CAD build for the part. Positions are in the model's coordinates, mm. A direction names the side the tool comes from. Give positions to 0.01 mm unless a question says otherwise; leave off trailing zeros. Loops run counter-clockwise (first coordinate to the right, second up) from the corner with the lowest first, then second, coordinate; pieces in that order, holes last. Notation, with made-up numbers: M 24,-14.5 L 28,-14.5 A25 ccw 28,13.5 Z; hole C 56.25,74.5 d4. An arc over 180 degrees is marked long. One line per question, with ' | ' between items.
```python
from build123d import *

# Parameters (mm, degrees)
BOSS_EXTRUDE1_DEPTH = 20
SKETCH5_W           = 9
SKETCH5_H           = 1.454272164
CUT_EXTRUDE4_DEPTH  = 10
SKETCH6_R           = 0.5
CUT_EXTRUDE5_DEPTH  = 5
CUT_EXTRUDE6_DEPTH  = 21
SKETCH11_R          = 1
CUT_EXTRUDE7_DEPTH  = 5


with BuildPart() as part:
    # Sketch1 → Boss-Extrude1 (new body)
    with BuildSketch(Plane.XY):
        with BuildLine():
            Line((0, 42.801960973), (0, -42.801960973))
            ThreePointArc((0, -42.801960973), (3.660110944, -50.535382386), (11.961161351, -52.60776773))
            Line((11.961161351, -52.60776773), (41.961161351, -46.60776773))
            ThreePointArc((41.961161351, -46.60776773), (47.733421413, -43.141850029), (50, -36.801960973))
            Line((50, -36.801960973), (50, 36.801960973))
            ThreePointArc((50, 36.801960973), (47.733421413, 43.141850029), (41.961161351, 46.60776773))
            Line((41.961161351, 46.60776773), (11.961161351, 52.60776773))
            ThreePointArc((11.961161351, 52.60776773), (3.660110944, 50.535382386), (0, 42.801960973))
        make_face()
    extrude(amount=BOSS_EXTRUDE1_DEPTH)

    # Sketch5 → Cut-Extrude4 (cut)
    with BuildSketch(Plane.ZY):
        with Locations((10, 16.569972364)):
            Rectangle(SKETCH5_W, SKETCH5_H)
    extrude(amount=-CUT_EXTRUDE4_DEPTH, mode=Mode.SUBTRACT)

    # Sketch6 → Cut-Extrude5 (cut)
    with BuildSketch(Plane.XZ.offset(-17.297108446)):
        with Locations((2.644871575, 10)):
            Circle(SKETCH6_R)
    extrude(amount=-CUT_EXTRUDE5_DEPTH, mode=Mode.SUBTRACT)

    # Sketch9 → Cut-Extrude6 (cut, through all)
    with BuildSketch(Plane.XY.offset(20)):
        Polygon((42.2, 5.497108446), (42.2, -10.402891554), (50, -10.402891554), (50, 12.297108446), (42.2, 12.297108446), (42.2, 7.997108446), (37.17, 7.997108446), (37.17, 5.497108446), align=None)
    extrude(amount=-CUT_EXTRUDE6_DEPTH, mode=Mode.SUBTRACT)

    # Sketch11 → Cut-Extrude7 (cut)
    with BuildSketch(Plane(origin=(0, 7.997108446, 0), x_dir=(-1, 0, 0), z_dir=(0, -1, 0))):
        with Locations((-39.9, -10)):
            Circle(SKETCH11_R)
    extrude(amount=-CUT_EXTRUDE7_DEPTH, mode=Mode.SUBTRACT)


solid = part.part
```
Item 1: Saw through at B-B on z = 17. Give the cut face in (x, y).
Conclusion:
outline: M 0,-42.8 A10 ccw 11.96,-52.61 L 41.96,-46.61 A10 ccw 50,-36.8 L 50,-10.4 L 42.2,-10.4 L 42.2,5.5 L 37.17,5.5 L 37.17,8 L 42.2,8 L 42.2,12.3 L 50,12.3 L 50,36.8 A10 ccw 41.96,46.61 L 11.96,52.61 A10 ccw 0,42.8 Z
Item 2: Drill centre lines: line 1 along Z through (x, y) = (39.9, 10.95); line 2 along X through (y, z) = (9.6, 10); line 3 along Y through (x, z) = (5.5, 11.25). Where is each one in solid material? Low to high. Write a range as [from, to].
Conclusion:
line 1: [0, 9], [11, 20] | line 2: [0, 38.9], [40.9, 42.2] | line 3: [-51.73, 15.84], [17.3, 51.73]
Item 3: Mould opens along Z. For faces 1 (the cylindrical face through (3.756, 50.613, 9.86)), 2 (the flat face through (25, 1, 0)), 3 (the cylindrical face through (40.637, 10.462, 9.324)) say: pulls with the +Z half, pulls with the -Z half, needs draft (parallel to the pull), parting line crosses it, or undercut.
Conclusion:
face 1: needs draft | face 2: pulls with the -Z half | face 3: undercut
Item 4: Saw through at A-A on x = 39.9. Give the cut face in (y, z), and give its area (3 significant figures).
Conclusion:
outline: M -47.02,0 L 5.5,0 L 5.5,20 L -47.02,20 Z; M 8,0 L 47.02,0 L 47.02,20 L 8,20 L 8,11 L 13,11 L 13,9 L 8,9 Z | area: 1,820 mm²
Item 5: Drop flat-ended pins along their axis: P1, Ø2.5, axis at x = 2.5, z = 11, coming from the -Y side; P2, Ø8, axis at x = 33, z = 13.5, coming from the -Y side; P3, Ø1, axis at x = 13, z = 6, coming from the +Y side. Give the stop position or say it passes through.
Conclusion:
P1: y = -50.61 | P2: y = -49.2 | P3: y = 52.5
Item 6: 3-axis set-ups, long thin cutter, end or side, ignore diameter. For faces 4 (the flat face through (40, 5.497, 10)), 5 (the flat face through (40, 12.997, 10)), 6 (the flat face through (27.171, 49.566, 9.86)), 7 (the flat face through (5, 15.843, 10)), 8 (the cylindrical face through (47.67, -43.22, 9.86)): which of +Z, -Z, +X, -X, +Y, -Y reach the whole face in a straight line?
Conclusion:
face 4: +Z, -Z, +X | face 5: none | face 6: +Z, -Z, +X, +Y | face 7: -X | face 8: +Z, -Z, +X, -Y
Item 7: Saw through at D-D on y = -9. Give the cut face in (x, z).
Conclusion:
outline: M 0,0 L 42.2,0 L 42.2,20 L 0,20 Z
Item 8: Saw through at C-C on x = 23. Give the cut face in (y, z), and give its area (3 significant figures).
Conclusion:
outline: M -50.4,0 L 50.4,0 L 50.4,20 L -50.4,20 Z | area: 2,020 mm²
